from build123d import *

# Parameters (mm, degrees)
SKETCH1_R           = 5.225
BOSS_EXTRUDE1_DEPTH = 6.5
BOSS_EXTRUDE1_TAPER = 1.5
DOME1_FACE_RADIUS   = 5.05479151
DOME1_HEIGHT        = 0.5
BOSS_EXTRUDE2_DEPTH = 2


# Read off the part's stored shape, not the designer's step: Shell1
with BuildPart() as part:
    # Sketch1 → Boss-Extrude1 (new body)
    with BuildSketch(Plane.XY):
        Circle(SKETCH1_R)
    extrude(amount=BOSS_EXTRUDE1_DEPTH, taper=BOSS_EXTRUDE1_TAPER)

    # Dome1: a dome of height H over a round flat face of radius A is a cap of a sphere of radius (A * A + H * H) / (2 * H)
    dome1_r = (DOME1_FACE_RADIUS * DOME1_FACE_RADIUS + DOME1_HEIGHT * DOME1_HEIGHT) / (2 * DOME1_HEIGHT)
    dome1_base = Plane((0, 0, 6.5), z_dir=(0, 0, 1))
    with Locations(dome1_base.offset(DOME1_HEIGHT - dome1_r)):
        dome1_ball = Sphere(dome1_r, mode=Mode.PRIVATE)
    add(split(dome1_ball, bisect_by=dome1_base, keep=Keep.TOP, mode=Mode.PRIVATE))

    # Shell1 outline → Shell1 (revolve, cut)
    with BuildSketch(Plane.XZ):
        with BuildLine():
            Line((3.474400113, 0), (3.343037716, 5.016528444))
            ThreePointArc((3.343037716, 5.016528444), (1.675590205, 5.191561114), (0, 5.25))
            Line((0, 5.25), (0, 0))
            Line((0, 0), (3.474400113, 0))
        make_face()
    revolve(axis=Axis((0, 0, 0), (0, 0, 1)), mode=Mode.SUBTRACT)

    # Sketch3 → Boss-Extrude2 (add)
    with BuildSketch(Plane(origin=(0, 0, 0), x_dir=(-1, 0, 0), z_dir=(0, 0, -1))):
        with BuildLine():
            Line((-6.875, 1), (-3.327379772, 1))
            ThreePointArc((-3.327379772, 1), (-3.474400113, 0), (-3.327379772, -1))
            Line((-3.327379772, -1), (-6.875, -1))
            ThreePointArc((-6.875, -1), (-7.875, 0), (-6.875, 1))
        make_face()
        with BuildLine():
            Line((3.327379772, 1), (6.875, 1))
            ThreePointArc((6.875, 1), (7.875, 0), (6.875, -1))
            Line((6.875, -1), (3.327379772, -1))
            ThreePointArc((3.327379772, -1), (3.474400113, 0), (3.327379772, 1))
        make_face()
    extrude(amount=-BOSS_EXTRUDE2_DEPTH)


solid = part.part
Geometry check sheet. Reference: the model listing, model coordinates, mm. Coordinates: 2 decimals unless noted, no trailing zeros. Loops run counter-clockwise (first coordinate to the right, second up) from the corner with the lowest first, then second, coordinate; pieces in that order, holes last. Notation, with made-up numbers: (66.5, 56.25) - (121.5, 56.25) arc R20 ccw to (121.5, 60.25) - close; hole circle Ø8 at (30.5, -0.5). An arc over 180 degrees is marked (long way). Use one line per item in the form item = value. Start each with the question number.
Item 1: Mould release check, pull along Y, two halves, no side actions. Record for faces 1 (the face through (4.901, 1.544, 3.296)), 2 (the face through (-4, 0, 0)), 3 (the face through (1.572, -3.023, 2.543)): +Y half, -Y half, draft (parallel to the pull), parting line (faces both ways), or undercut.
Item 2: Section check C-C, the plane z = 1.5. Enter the section's corners in (x, y) (3 decimals), and give its area (3 significant figures).
Item 3: Gauge pin test, flat ends, axial feed: pin 1 (0.5 mm diameter, centred on x = -6.5, z = 1, fed in from -Y); pin 2 (0.6 mm diameter, centred on x = 7, y = 0, fed in from +Z); pin 3 (3 mm diameter, centred on x = -3, y = -0.5, fed in from +Z). Record the tip position at first contact, or that the pin passes through.
Item 4: Section check B-B, the plane x = 0. Enter the section's corners in (y, z) (3 decimals), and give its area (3 significant figures).
Item 5: Section check D-D, the plane z = 4.75. Enter the section's corners in (x, y), and give its area (3 significant figures).
Item 6: Thickness scan on probe 1 along Y at (x, z) = (1, 2); probe 2 along Y at (x, z) = (-2.75, 4.5); probe 3 along X at (y, z) = (-0.25, 4.5). Record the ranges inside material, lowest first.
Item 7: Section check A-A, the plane y = 0. Enter the section's corners in (x, z) (3 decimals).
Computed:
q1.face_1 = parting line
q1.face_2 = draft
q1.face_3 = undercut
q2.outline = (-6.875, -1) - (-5.088, -1) arc R5.186 ccw to (5.088, -1) - (6.875, -1) arc R1 ccw to (6.875, 1) - (5.088, 1) arc R5.186 ccw to (-5.088, 1) - (-6.875, 1) arc R1 ccw to start; hole circle Ø6.87 at (0, 0)
q2.area = 57.4 mm2
q3.pin_1 = -1
q3.pin_2 = 2
q3.pin_3 = 6.95
q4.outline = (-5.225, 0) - (-3.474, 0) - (-3.343, 5.017) arc R24.051 cw to (3.343, 5.017) - (3.474, 0) - (5.225, 0) - (5.055, 6.5) arc R25.801 ccw to (-5.055, 6.5) - close
q4.area = 35.0 mm2
q5.outline = circle Ø10.2 at (0, 0); hole circle Ø6.7 at (0, 0)
q5.area = 46.5 mm2
q6.probe_1 = -5.08 to -3.27, 3.27 to 5.08
q6.probe_2 = -4.3 to -1.92, 1.92 to 4.3
q6.probe_3 = -5.1 to -3.35, 3.35 to 5.1
q7.outline = (-7.875, 0) - (-3.474, 0) - (-3.343, 5.017) arc R24.051 cw to (3.343, 5.017) - (3.474, 0) - (7.875, 0) - (7.875, 2) - (5.173, 2) - (5.055, 6.5) arc R25.801 ccw to (-5.055, 6.5) - (-5.173, 2) - (-7.875, 2) - close
